from build123d import *

# Parameters (mm, degrees)
SKETCH1_R                 = 1
BOSS_EXTRUDE_8_10MM_DEPTH = 8.1
F_0_5_X_45_DEG_SIZE       = 0.5


with BuildPart() as part:
    # Sketch1 → Boss-Extrude 8.10mm (new body)
    with BuildSketch(Plane(origin=(0, 0, 0), x_dir=(1, 0, 0), z_dir=(0, 1, 0))):
        Circle(SKETCH1_R)
    extrude(amount=-BOSS_EXTRUDE_8_10MM_DEPTH)

    # 0.5 x 45 deg
    f_0_5_x_45_deg_edges = [part.edges().sort_by_distance(p)[0] for p in [
        (-1, -8.1, 0),
    ]]
    chamfer(f_0_5_x_45_deg_edges, length=F_0_5_X_45_DEG_SIZE)

    # Sketch2 → SR8 (revolve, cut)
    with BuildSketch(Plane.XY):
        with BuildLine():
            Line((0, 2), (-2, 2))
            Line((-2, 2), (-2, -0.254033308))
            ThreePointArc((-2, -0.254033308), (-1.00803434, -0.06376243), (0, 0))
            Line((0, 0), (0, 2))
        make_face()
    revolve(axis=Axis((0, 0, 0), (0, 1, 0)), mode=Mode.SUBTRACT)


solid = part.part
Model file for the job. Use its own axes, mm. Coordinates: 2 decimals unless noted, no trailing zeros. Order: outer loops, then holes, each group sorted by start corner. A loop starts at its lowest first (then second) coordinate and runs counter-clockwise, first axis right, second up. Notation, with made-up numbers: (22.5, 39) -> (78.5, 39) arc R20 cw to (78.5, 77) -> close; hole circle Ø5 at (49, -20.5). An arc over 180 degrees is marked (long way). Return JSON: item names as keys, results as strings. Group by question number.
Item 1: Saw through at C-C on y = -6.5. Write the cut outline in (x, z).
Item 2: Saw through at A-A on z = 0. Write the cut outline in (x, y), then the cut area to 3 significant figures.
Item 3: Saw through at B-B on x = 0. Write the cut outline in (y, z).
Item 4: Wall check: line 1 along Y through (x, z) = (0.15, 0.1); line 2 along X through (y, z) = (-4.75, 0.2); line 3 along X through (y, z) = (-5, -0.6). Give the ranges that are in metal, low to high. Write a range as [from, to].
Item 5: Flat gauge pin, fed straight in: P1, Ø1, axis at x = 0.5, z = -0.5, coming from the -Y side. Where does the tip first touch, or does it go through?
Values found:
{
 "1": {"outline": "circle Ø2 at (0, 0)"},
 "2": {"outline": "(-1, -7.6) -> (-0.5, -8.1) -> (0.5, -8.1) -> (1, -7.6) -> (1, -0.06) arc R8 ccw to (-1, -0.06) -> close", "area": "15.9 mm2"},
 "3": {"outline": "(-8.1, -0.5) -> (-7.6, -1) -> (-0.06, -1) arc R8 ccw to (-0.06, 1) -> (-7.6, 1) -> (-8.1, 0.5) -> close"},
 "4": {"line 1": "y = [-8.1, 0]", "line 2": "x = [-0.98, 0.98]", "line 3": "x = [-0.8, 0.8]"},
 "5": {"P1": "stops at y = -8.1"}
}
